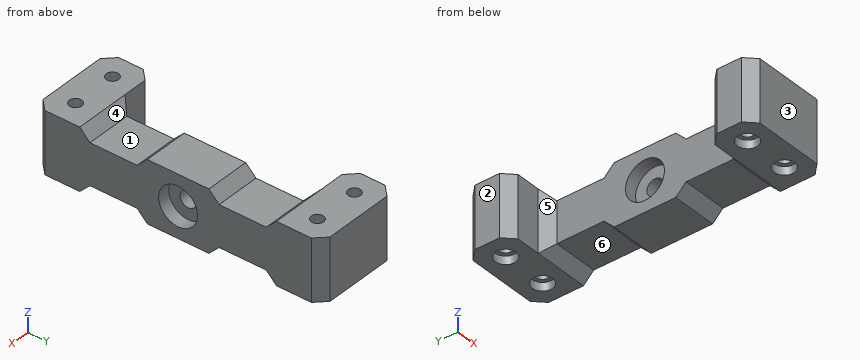
Autodesk Inventor part; units mm, degrees
ref_plane "YZ Plane" through (0, 0, 0) normal (1, 0, 0) x (0, 1, 0)
ref_plane "XZ Plane" through (0, 0, 0) normal (0, 1, 0) x (-1, 0, 0)
ref_plane "XY Plane" through (0, 0, 0) normal (0, 0, 1) x (1, 0, 0)
sketch "Esquisse17" plane through (0, 0, 0) normal (0, 0, 1) x (1, 0, 0)
  line L0 (-22, 70) -> (22, 70)
  line L1 (22, 70) -> (22, -70)
  line L2 (22, -70) -> (-22, -70)
  line L3 (-22, -70) -> (-22, 70)
  point P0 (0, 0)
  dimension "d107" = 70
  dimension "d108" = 140
  dimension "d109" = 44
  dimension "d110" = 22
extrude "Extrusion13" add sketch "Esquisse17" along normal mid plane 30
sketch "Esquisse18" plane through (22, -70, 15) normal (1, 0, 0) x (0, 0, -1)
  circle A0 centre (15, 70) radius 4
  dimension "d113" = 8
extrude "Extrusion14" cut sketch "Esquisse18" against normal up to next
sketch "Esquisse19" plane through (22, -70, 15) normal (1, 0, 0) x (0, 0, -1)
  circle A0 centre (15, 70) radius 9.5
  dimension "d116" = 19
extrude "Extrusion15" cut sketch "Esquisse19" against normal blind 6
sketch "Esquisse20" plane through (0, 0, 15) normal (0, 0, 1) x (1, 0, 0)
  line L0 (-22, 48) -> (0, 48)
  line L1 (0, 48) -> (0, -48)
  line L2 (0, -48) -> (-22, -48)
  line L3 (-22, -48) -> (-22, 48)
  line L4 (22, -70) -> (22, 70)
  line L5 (-22, 70) -> (-22, -70)
  point P0 (0, 0)
  dimension "d119" = 96
  dimension "d120" = 48
  dimension "d121" = 22
extrude "Extrusion16" cut sketch "Esquisse20" against normal up to next
sketch "Esquisse21" plane through (0, -48, 15) normal (-1, 0, 0) x (0, 0, 1)
  circle A0 centre (-15, 48) radius 9.5
  dimension "d125" = 19
extrude "Extrusion17" cut sketch "Esquisse21" against normal blind 6
sketch "Esquisse22" plane through (22, -70, 15) normal (1, 0, 0) x (0, 0, -1)
  line L0 (5, 0) -> (25, 0)
  line L1 (25, 140) -> (5, 140)
  line L2 (0, 0) -> (30, 0)
  line L3 (0, 140) -> (30, 140)
  line L4 (0, 0) -> (0, 140)
  line L5 (30, 140) -> (30, 0)
  line L6 (30, 55) -> (30, 85)
  line L7 (0, 85) -> (0, 55)
  line L8 (0, 55) -> (0, 55)
  line L9 (30, 55) -> (30, 55)
  line L10 (5, 140) -> (5, 90)
  line L11 (5, 50) -> (5, 0)
  line L12 (25, 0) -> (25, 50)
  line L13 (25, 90) -> (25, 140)
  line L14 (30, 85) -> (30, 85)
  line L15 (0, 85) -> (0, 85)
  line L16 (0, 55) -> (5, 50)
  line L17 (5, 90) -> (0, 85)
  line L18 (25, 90) -> (30, 85)
  line L19 (30, 55) -> (25, 50)
  line L20 (0, 118) -> (5, 118)
  line L21 (25, 118) -> (30, 118)
  line L22 (0, 22) -> (5, 22)
  line L23 (25, 22) -> (30, 22)
  point P0 (15, 70)
  point P1 (5, 55)
  point P2 (25, 55)
  point P3 (5, 85)
  point P4 (25, 85)
  dimension "d131" = 30
  dimension "d133" = 20
  dimension "d134" = 10
  dimension "d135" = 30
  dimension "d136" = 15
  dimension "d137" = 5
  dimension "d138" = 5
  dimension "d139" = 5
  dimension "d140" = 5
  dimension "d141" = 5
  dimension "d142" = 5
  dimension "d143" = 5
  dimension "d144" = 5
extrude "Extrusion19" cut sketch "Esquisse22" against normal up to next contours L22 L4 L16 L11 | L12 L19 L5 L23 | L4 L20 L10 L17 | L18 L13 L21 L5
chamfer "Chanfrein3" distance 5 angle 45 10 edges at (11, -48, -10) (11, -48, 10) (11, 48, 10) (11, 48, -10) (-22, -48, 0) (-22, -70, 0) (-22, 48, 0) (-22, 70, 0) (22, -70, 0) (22, 70, 0)
sketch "Esquisse23" plane through (0, 0, -15) normal (0, 0, -1) x (-1, 0, 0)
  line L0 (-11, -59) -> (11, -59)
  line L1 (17, -48) -> (0, -48)
  line L2 (0, -48) -> (-22, -48)
  line L3 (-22, -48) -> (-22, -65)
  line L4 (-17, -70) -> (17, -70)
  line L5 (22, -65) -> (22, -53)
  line L6 (-46.7579, 0) -> (65.4048, 0)
  line L7 (-11, 59) -> (11, 59)
  line L8 (20, 48) -> (0, 48)
  line L9 (0, 48) -> (-22, 48)
  line L10 (-22, 48) -> (-22, 70)
  line L11 (-22, 70) -> (20, 70)
  line L12 (20, 70) -> (20, 48)
  line L13 (0, 15) -> (-22, 15)
  line L14 (-22, 15) -> (-22, -15)
  line L15 (-22, -15) -> (0, -15)
  line L16 (0, -15) -> (0, 15)
  line L17 (-17, -70) -> (-22, -65)
  line L18 (22, -65) -> (17, -70)
  line L19 (17, -48) -> (22, -53)
  line L20 (-22, 65) -> (-17, 70)
  line L21 (-22, 48) -> (0, 48)
  line L22 (0, 48) -> (17, 48)
  line L23 (22, 53) -> (17, 48)
  line L24 (22, 53) -> (22, 65)
  line L25 (17, 70) -> (22, 65)
  line L26 (17, 70) -> (-17, 70)
  line L27 (-22, 65) -> (-22, 48)
  point P0 (0, 0)
  dimension "d153" = 11
  dimension "d154" = 11
  dimension "d155" = 11
hole "Perçage4" at (11, -59, -15) at (-11, -59, -15) at (11, 59, -15) at (-11, 59, -15) direction (0, 0, 1) diameter 6 end through all counterbore diameter 10 counterbore depth 4
chamfer "Chanfrein4" distance 5 angle 45 2 edges at (0, 48, 0) (0, -48, 0)
equation "\"d135\" = d131"
equation "\"d153\" = 0.5 * d152"
equation "\"d154\" = d153"
equation "\"d155\" = d153"
equation "\"d132\" = 0.5 * d130"
properties part number "Wheel_Block"
Here's how the part is built. I have some questions about the finished solid (model axes, mm). Face numbers are marked on the shaded views. A direction names the side the tool comes from. Give positions to 0.01 mm unless a question says otherwise; leave off trailing zeros. Loops run counter-clockwise (first coordinate to the right, second up) from the corner with the lowest first, then second, coordinate; pieces in that order, holes last. Notation, with made-up numbers: (10.25, -23) -> (17.25, -23) arc R26 ccw to (17.25, 14) -> close; hole circle Ø5 at (31.25, 43). An arc over 180 degrees is marked (long way). Use one line per item in the form item = value. Start each with the question number.
1) Imagine slicing it at D-D (y = 0). Please give me the cut outline in (x, z).
2) Imagine slicing it at A-A (z = 0). Count the separate pieces of the cut face and the enclosed holes in it, then the cut area to 3 significant figures.
3) Please list where these lines run through material, in increasing order: line 1 along X through (y, z) = (59, 4.75); line 2 along X through (y, z) = (-59, -12.3); line 3 along Y through (x, z) = (-11, 8).
4) For P1, Ø6.5, axis at x = 15, y = -36, coming from the -Z side; P2, Ø9, axis at y = 0, z = 0, coming from the +X side; P3, Ø10, axis at y = -6.5, z = 8.5, coming from the -X side, each with a flat end and sliding along its axis, tell me the tip position at first contact or that it passes through.
5) Imagine slicing it at C-C (y = -59). Please give me the cut outline in (x, z), then the cut area to 3 significant figures.
6) Which directions (+Z, -Z, +X, -X, +Y, -Y) give clear straight access to the entire face, cutting with the end or side of a thin tool? Please do the marked faces 4, 5 and 6.
7) Imagine slicing it at B-B (x = -11). Please give me the cut outline in (y, z), then the cut area to 3 significant figures.
8) Thinking about a two-plate mould opening in Y: for the marked faces 1, 2 and 3, which applies, +Y half, -Y half, draft (parallel to the pull), parting line (faces both ways), or undercut?
Check values:
q1.outline = (0, -15) -> (22, -15) -> (22, -9.5) -> (16, -9.5) -> (16, -4) -> (6, -4) -> (6, -9.5) -> (0, -9.5) -> close; (0, 9.5) -> (6, 9.5) -> (6, 4) -> (16, 4) -> (16, 9.5) -> (22, 9.5) -> (22, 15) -> (0, 15) -> close
q2.separate_pieces = 2
q2.enclosed_holes = 4
q2.area = 3,580 mm^2
q3.line_1 = -22 to -14, -8 to 8, 14 to 22
q3.line_2 = -22 to -16, -6 to 6, 16 to 22
q3.line_3 = -70 to -62, -56 to -48, 48 to 56, 62 to 70
q4.P1 = -10
q4.P2 = 16
q4.P3 = 0
q5.outline = (-22, -15) -> (-16, -15) -> (-16, -11) -> (-14, -11) -> (-14, 15) -> (-22, 15) -> close; (-8, -11) -> (-6, -11) -> (-6, -15) -> (6, -15) -> (6, -11) -> (8, -11) -> (8, 15) -> (-8, 15) -> close; (14, -11) -> (16, -11) -> (16, -15) -> (22, -15) -> (22, 15) -> (14, 15) -> close
q5.area = 928 mm^2
q6.face_4 = +Z, +X, -X
q6.face_5 = +Z, -Z, -X
q6.face_6 = -Z, +X, -X
q7.outline = (-70, -15) -> (-64, -15) -> (-64, -11) -> (-62, -11) -> (-62, 15) -> (-70, 15) -> close; (-56, -11) -> (-54, -11) -> (-54, -15) -> (-48, -15) -> (-48, 15) -> (-56, 15) -> close; (48, -15) -> (54, -15) -> (54, -11) -> (56, -11) -> (56, 15) -> (48, 15) -> close; (62, -11) -> (64, -11) -> (64, -15) -> (70, -15) -> (70, 15) -> (62, 15) -> close
q7.area = 928 mm^2
q8.face_1 = undercut
q8.face_2 = draft
q8.face_3 = -Y half
